Input: part model. Units: mm. Frame: model coordinates. A direction names the side the tool comes from. Give positions to 0.01 mm unless a question says otherwise; leave off trailing zeros. Loops run counter-clockwise (first coordinate to the right, second up) from the corner with the lowest first, then second, coordinate; pieces in that order, holes last. Notation, with made-up numbers: (34, 22.25) - (42, 22.25) arc R13 cw to (42, 43.25) - close; hole circle Ø3 at (-30, 22.5). An arc over 180 degrees is marked (long way). Answer as a JSON object with one key per item and string values. Group by question number.
(1) Access query for faces 4 (the flat face through (80.014, -0.441, 21.756)), 5 (the flat face through (18, 2.5, 43)), 6 (the flat face through (-19, 10, 16)). Directions: +Z, -Z, +X, -X, +Y, -Y. A direction counts if a zero-diameter tool reaches every point of the face in a straight line with its end or side. Return the directions, or none.
(2) Pin query (flat end, axial travel): P1, Ø1.3, axis at x = 23.5, z = 43.5, coming from the +Y side; P2, Ø3, axis at x = 26, z = 34.5, coming from the -Y side; P3, Ø8, axis at x = 11, z = 35, coming from the -Y side. Return the tip coordinate at first contact, or that it passes through.
(3) Section query A-A (x = 31). Return loops of the section in (y, z), plus the area to 3 significant figures.
(4) Mould query, pull axis Y, two halves, no side actions, for faces 1 (the flat face through (-18, 0, 7.3)), 2 (the flat face through (49, -1.5, 41)), 3 (the flat face through (-18, -5, 10)). Classes: +Y half, -Y half, draft (parallel to the pull), parting line (faces both ways), or undercut.
(5) Material intervals for L1, parallel to Y at x = 65.5, z = 14.5; L2, parallel to Y at x = 26, z = 39; L3, parallel to X at y = 6.5, z = 14, sorted ascending.
(6) Section query C-C (z = 32.5). Return loops of the section in (x, y), plus the area to 3 significant figures.
(7) Section query D-D (x = 10). Return loops of the section in (y, z), plus the area to 3 significant figures.
(8) Section query B-B (y = 6.5). Return loops of the section in (x, z).
```python
from build123d import *

# Parameters (mm, degrees)
PAD003_DEPTH    = 33.5
SKETCH015_W     = 120
SKETCH015_H     = 100
POCKET011_DEPTH = 123.001
THICKNESS_T     = -2
PAD004_DEPTH    = 31.5
POCKET012_DEPTH = 13
PAD005_DEPTH    = 10
PAD006_DEPTH    = 5
PAD007_DEPTH    = 2
POCKET013_DEPTH = 5
CHAMFER001_SIZE = 1


with BuildPart() as part:
    # Sketch014 → Pad003 (new body, symmetric)
    with BuildSketch(Plane.XZ):
        Polygon((-23, 23.5), (0, 45), (79, 39), (83, 28.5), (83, 13.5), (-23, 13.5), align=None)
    extrude(amount=PAD003_DEPTH, both=True)

    # Sketch015 (on DatumPlane) → Pocket011 (cut, through all)
    with BuildSketch(Plane.YZ.offset(100)):
        with Locations((0, 16.75)):
            Rectangle(SKETCH015_W, SKETCH015_H)
        Polygon((-33.5, 27.5), (-7.25, 53.75), (7.25, 53.75), (33.5, 27.5), (33.5, 13.5), (-33.5, 13.5), align=None, mode=Mode.SUBTRACT)
    extrude(amount=-POCKET011_DEPTH, mode=Mode.SUBTRACT)

    # Thickness
    thickness_openings = [part.faces().sort_by_distance(p)[0] for p in [
        (30, 0, 13.5),
    ]]
    offset(amount=THICKNESS_T, openings=thickness_openings)

    # Sketch020 (on DatumPlane) → Pad004 (join, symmetric)
    with BuildSketch(Plane.XZ):
        Polygon((83, 26.928203), (79, 20), (79, 13.5), (83, 13.5), align=None)
    extrude(amount=PAD004_DEPTH, both=True)

    # Sketch021 (on DatumPlane) → Pocket012 (cut, symmetric)
    with BuildSketch(Plane.XZ):
        Polygon((78.817394, 18.7), (81.3, 18.7), (78.817394, 14.4), align=None)
    extrude(amount=POCKET012_DEPTH, both=True, mode=Mode.SUBTRACT)

    # Sketch022 (on DatumPlane) → Pad005 (join, symmetric)
    with BuildSketch(Plane.XZ):
        Polygon((-21, 20.947818), (-16.7, 13.5), (-16.7, 12.5), (-18.7, 12.5), (-18.7, 13.5), (-21, 13.5), align=None)
    extrude(amount=PAD005_DEPTH, both=True)

    # Sketch023 (on DatumPlane) → Pad006 (join, symmetric)
    with BuildSketch(Plane.XZ):
        Polygon((-18.7, 13.5), (-18.7, 12.5), (-20.8, 10.4), (-20.8, 9.4), (-18.7, 7.3), (-16.7, 7.3), (-16.7, 13.5), align=None)
    extrude(amount=PAD006_DEPTH, both=True)

    # Sketch024 (on Face6 of Pad006) → Pad007 (join)
    with BuildSketch(Plane.XZ.offset(33.5)):
        Polygon((55.2, 13.5), (47.003848, 13.5), (52.2, 10.5), (55.2, 10.5), align=None)
    pad007 = extrude(amount=-PAD007_DEPTH)

    # Mirrored004: Pad007 across XZ
    add(pad007.mirror(Plane.XZ))

    # Sketch025 (on DatumPlane) → Pocket013 (cut)
    with BuildSketch(Plane(origin=(3.39812, 0, 44.741915), x_dir=(0.997128, 0, -0.075731), z_dir=(0.075731, 0, 0.997128))):
        Polygon((0, 2.5), (30, 2.5), (31, 1.5), (61, 1.5), (61, -1.5), (31, -1.5), (30, -2.5), (0, -2.5), align=None)
    extrude(amount=-POCKET013_DEPTH, mode=Mode.SUBTRACT)

    # Chamfer001
    chamfer001_edges = [part.edges().sort_by_distance(p)[0] for p in [
        (49.114558, 1.5, 39.26402),
        (49.114558, -1.5, 39.26402),
    ]]
    chamfer(chamfer001_edges, length=CHAMFER001_SIZE)


solid = part.part
```
Recorded:
{
 "1": {"face 4": "none", "face 5": "+Z, -Z", "face 6": "-Z"},
 "2": {"P1": "stops at y = 18.15", "P2": "stops at y = -28", "P3": "stops at y = -30"},
 "3": {"outline": "(-33.5, 13.5) - (-31.5, 13.5) - (-31.5, 26.67) - (-17.53, 40.64) - (-2.5, 40.64) - (-2.5, 42.65) - (-18.35, 42.65) - (-33.5, 27.5) - close; (2.5, 40.64) - (17.53, 40.64) - (31.5, 26.67) - (31.5, 13.5) - (33.5, 13.5) - (33.5, 27.5) - (18.35, 42.65) - (2.5, 42.65) - close", "area": "199 mm^2"},
 "4": {"face 1": "draft", "face 2": "undercut", "face 3": "-Y half"},
 "5": {"L1": "y = -33.5 to -31.5, 31.5 to 33.5", "L2": "y = -22 to -19.17, 19.17 to 22", "L3": "x = -23 to -16.99, 79 to 83"},
 "6": {"outline": "(-13.37, -28.5) - (81.48, -28.5) - (81.48, 28.5) - (-13.37, 28.5) - close; hole (-10.44, -25.67) - (79.34, -25.67) - (79.34, 25.67) - (-10.44, 25.67) - close", "area": "797 mm^2"},
 "7": {"outline": "(-33.5, 13.5) - (-31.5, 13.5) - (-31.5, 26.67) - (-15.94, 42.23) - (-2.5, 42.23) - (-2.5, 44.24) - (-16.76, 44.24) - (-33.5, 27.5) - close; (2.5, 42.23) - (15.94, 42.23) - (31.5, 26.67) - (31.5, 13.5) - (33.5, 13.5) - (33.5, 27.5) - (16.76, 44.24) - (2.5, 44.24) - close", "area": "201 mm^2"},
 "8": {"outline": "(-23, 13.5) - (-18.7, 13.5) - (-18.7, 12.5) - (-16.7, 12.5) - (-16.7, 13.5) - (-21, 20.95) - (-21, 22.63) - (0.72, 42.94) - (77.58, 37.1) - (81, 28.13) - (81, 23.46) - (79, 20) - (79, 18.7) - (81.3, 18.7) - (79, 14.72) - (79, 13.5) - (83, 13.5) - (83, 28.5) - (79, 39) - (0, 45) - (-23, 23.5) - close"}
}
